```python
from build123d import *

# Parameters (mm, degrees)
SKETCH1_W           = 60
SKETCH1_H           = 110
BOSS_EXTRUDE1_DEPTH = 3
SKETCH2_R           = 1.55
CUT_EXTRUDE1_DEPTH  = 3
CUT_EXTRUDE2_DEPTH  = 2.33
CUT_EXTRUDE3_DEPTH  = 0.67
BOSS_EXTRUDE3_DEPTH = 25
SKETCH9_W           = 45
SKETCH9_H           = 6.8
BOSS_EXTRUDE4_DEPTH = 2
SKETCH10_W          = 5.4
SKETCH10_H          = 6.8
BOSS_EXTRUDE5_DEPTH = 14.5
FILLET1_R           = 2.5
SKETCH11_R          = 0.75
BOSS_EXTRUDE6_DEPTH = 6
SKETCH12_W          = 1.2
SKETCH12_H          = 0.8
CUT_EXTRUDE4_DEPTH  = 0.1


with BuildPart() as part:
    # Sketch1 → Boss-Extrude1 (new body)
    with BuildSketch(Plane(origin=(0, 0, 0), x_dir=(1, 0, 0), z_dir=(0, 1, 0))):
        with Locations((30, 55)):
            Rectangle(SKETCH1_W, SKETCH1_H)
    extrude(amount=BOSS_EXTRUDE1_DEPTH)

    # Sketch2 → Cut-Extrude1 (cut)
    with BuildSketch(Plane(origin=(0, 3, 0), x_dir=(1, 0, 0), z_dir=(0, 1, 0))):
        with Locations(Location((7.5, 7.5, 0), (0, 0, 270))):
            Circle(SKETCH2_R)
        with Locations(Location((52.5, 7.5, 0), (0, 0, 270))):
            Circle(SKETCH2_R)
        with Locations(Location((7.5, 72.5, 0), (0, 0, 270))):
            Circle(SKETCH2_R)
        with Locations(Location((52.5, 72.5, 0), (0, 0, 270))):
            Circle(SKETCH2_R)
    extrude(amount=-CUT_EXTRUDE1_DEPTH, mode=Mode.SUBTRACT)

    # Sketch3 → Cut-Extrude2 (cut)
    with BuildSketch(Plane(origin=(0, 3, 0), x_dir=(1, 0, 0), z_dir=(0, 1, 0))):
        with BuildLine():
            Line((35, 33.1), (35, 30))
            ThreePointArc((35, 30), (30, 25), (25, 30))
            Line((25, 30), (25, 33.1))
            ThreePointArc((25, 33.1), (30, 38.1), (35, 33.1))
        make_face()
    extrude(amount=-CUT_EXTRUDE2_DEPTH, mode=Mode.SUBTRACT)

    # Sketch4 → Cut-Extrude3 (cut)
    with BuildSketch(Plane.XZ):
        with BuildLine():
            Line((26.98, -20.051339235), (33.02, -20.051339235))
            ThreePointArc((33.02, -20.051339235), (38.181879503, -22.189459733), (40.32, -27.351339235))
            Line((40.32, -27.351339235), (40.32, -35.65))
            ThreePointArc((40.32, -35.65), (38.181879503, -40.811879503), (33.02, -42.95))
            Line((33.02, -42.95), (26.980030862, -42.930691587))
            ThreePointArc((26.980030862, -42.930691587), (21.840512337, -40.791632856), (19.703396192, -35.65130626))
            Line((19.703396192, -35.65130626), (19.68, -27.351339235))
            ThreePointArc((19.68, -27.351339235), (21.818120497, -22.189459733), (26.98, -20.051339235))
        make_face()
    extrude(amount=-CUT_EXTRUDE3_DEPTH, mode=Mode.SUBTRACT)

    # Sketch6 → Boss-Extrude3 (add)
    with BuildSketch(Plane.XZ):
        Polygon((51.3, -93.2), (52.5, -93.2), (52.5, -88.2), (47.1, -88.2), (47.1, -93.2), (48.3, -93.2), (48.3, -94), (47.1, -94), (47.1, -95), (52.5, -95), (52.5, -94), (51.3, -94), align=None)
        Polygon((11.7, -93.2), (12.9, -93.2), (12.9, -88.2), (7.5, -88.2), (7.5, -93.2), (8.7, -93.2), (8.7, -94), (7.5, -94), (7.5, -95), (12.9, -95), (12.9, -94), (11.7, -94), align=None)
    extrude(amount=BOSS_EXTRUDE3_DEPTH)

    # Sketch9 → Boss-Extrude4 (add)
    with BuildSketch(Plane(origin=(0, -16.5, 0), x_dir=(1, 0, 0), z_dir=(0, 1, 0))):
        with Locations((30, 91.6)):
            Rectangle(SKETCH9_W, SKETCH9_H)
    extrude(amount=BOSS_EXTRUDE4_DEPTH)

    # Sketch10 → Boss-Extrude5 (add)
    with BuildSketch(Plane.XZ):
        with Locations((10.2, -91.6)):
            Rectangle(SKETCH10_W, SKETCH10_H)
        with Locations((49.8, -91.6)):
            Rectangle(SKETCH10_W, SKETCH10_H)
    extrude(amount=BOSS_EXTRUDE5_DEPTH)

    # Fillet1
    fillet1_edges = [part.edges().sort_by_distance(p)[0] for p in [
        (0, 1.5, -110),
        (60, 1.5, -110),
        (60, 1.5, 0),
        (0, 1.5, 0),
    ]]
    fillet(fillet1_edges, radius=FILLET1_R)

    # Sketch11 → Boss-Extrude6 (add)
    with BuildSketch(Plane.XZ):
        with Locations(Location((30, -18.551339235, 0), (0, 0, 270))):
            Circle(SKETCH11_R)
        with Locations(Location((30, -44.940355963, 0), (0, 0, 270))):
            Circle(SKETCH11_R)
    extrude(amount=BOSS_EXTRUDE6_DEPTH)

    # Sketch12 → Cut-Extrude4 (cut)
    with BuildSketch(Plane.XZ.offset(16.5)):
        Polygon((12.9, -94), (12.9, -95), (47.1, -95), (47.1, -94), (48.3, -94), (48.3, -93.2), (47.1, -93.2), (47.1, -88.2), (12.9, -88.2), (12.9, -93.2), (11.7, -93.2), (11.7, -94), align=None)
        with Locations((8.1, -93.6)):
            Rectangle(SKETCH12_W, SKETCH12_H)
        with Locations((51.9, -93.6)):
            Rectangle(SKETCH12_W, SKETCH12_H)
    extrude(amount=-CUT_EXTRUDE4_DEPTH, mode=Mode.SUBTRACT)


solid = part.part
```
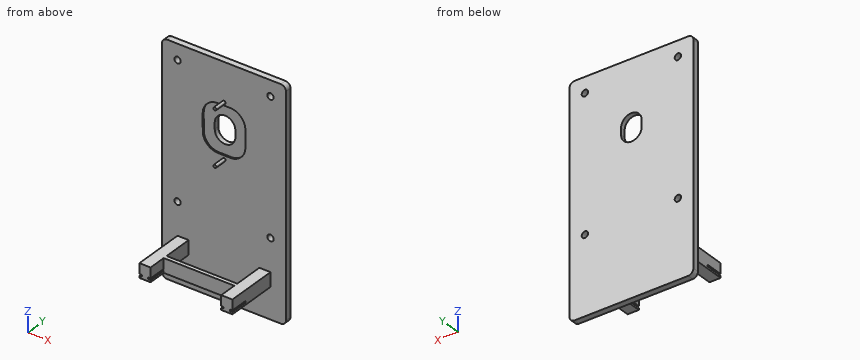
Can you work these out from the model? Positions are in its coordinate system, mm. Round coordinates to 2 decimals unless told otherwise and drop trailing zeros. Loops run counter-clockwise (first coordinate to the right, second up) from the corner with the lowest first, then second, coordinate; pieces in that order, holes last. Notation, with made-up numbers: M 73.5,-0.5 L 121.5,-0.5 A31 cw 121.5,32.5 Z; hole C -22,21 d10. An arc over 180 degrees is marked long. Write item = value, one per line. Start each with the question number.
(1) I need wall thicknesses on line 1 along X through (y, z) = (0.8, -72.5); line 2 along X through (y, z) = (-22, -91.5); line 3 along Y through (x, z) = (31, -6.5). Which ranges of each line are inside material? Lowest first, please.
(2) Suppose I cut it at C-C on x = 15.5. Write out the boundary of the cut face in (y, z), plus the area to 3 significant figures.
(3) Suppose I cut it at D-D on y = -2. Write out the boundary of the cut face in (x, z), plus the area to 3 significant figures.
(4) Suppose I cut it at A-A on z = -7.5. Write out the boundary of the cut face in (x, y), plus the area to 3 significant figures.
(5) I'm going to push flat-ended pins straight in: P1, Ø1.6, axis at x = 30, z = -18.5, coming from the -Y side; P2, Ø6, axis at x = 25, y = -7.5, coming from the -Z side; P3, Ø3.5, axis at y = -7.5, z = -93, coming from the +X side; P4, Ø8, axis at x = 39, y = -15, coming from the +Z side. Where does each tip first touch, or does it pass through?
(6) Suppose I cut it at B-B on y = -22.5. Write out the boundary of the cut face in (x, z), plus the area to 3 significant figures.
Answer block:
q1.line_1 = 0 to 5.95, 9.05 to 50.95, 54.05 to 60
q1.line_2 = 7.5 to 12.9, 47.1 to 52.5
q1.line_3 = 0 to 3
q2.outline = M -16.4,-95 L -14.5,-95 L -14.5,-88.2 L -16.4,-88.2 Z; M 0,-110 L 3,-110 L 3,0 L 0,0 Z
q2.area = 343 mm²
q3.outline = M 7.5,-95 L 12.9,-95 L 12.9,-88.2 L 7.5,-88.2 Z; C 30,-44.94 d1.5; C 30,-18.55 d1.5; M 47.1,-95 L 52.5,-95 L 52.5,-88.2 L 47.1,-88.2 Z
q3.area = 77.0 mm²
q4.outline = M 0,0 L 5.95,0 L 5.95,3 L 0,3 Z; M 9.05,0 L 50.95,0 L 50.95,3 L 9.05,3 Z; M 54.05,0 L 60,0 L 60,3 L 54.05,3 Z
q4.area = 161 mm²
q5.P1 = -6
q5.P2 = through
q5.P3 = 52.5
q5.P4 = -88.2
q6.outline = M 7.5,-95 L 12.9,-95 L 12.9,-94 L 11.7,-94 L 11.7,-93.2 L 12.9,-93.2 L 12.9,-88.2 L 7.5,-88.2 L 7.5,-93.2 L 8.7,-93.2 L 8.7,-94 L 7.5,-94 Z; M 47.1,-95 L 52.5,-95 L 52.5,-94 L 51.3,-94 L 51.3,-93.2 L 52.5,-93.2 L 52.5,-88.2 L 47.1,-88.2 L 47.1,-93.2 L 48.3,-93.2 L 48.3,-94 L 47.1,-94 Z
q6.area = 69.6 mm²
